Could you check a few things on this model? Use its own coordinates, in mm. Face numbers are marked on the shaded views. A direction names the side the tool comes from. Round coordinates to 2 decimals unless told otherwise and drop trailing zeros. Loops run counter-clockwise (first coordinate to the right, second up) from the corner with the lowest first, then second, coordinate; pieces in that order, holes last. Notation, with made-up numbers: (59.5, -22.75) - (65.5, -22.75) arc R17 ccw to (65.5, 1.25) - close; hole circle Ø5 at (-5, 82.5). An arc over 180 degrees is marked (long way). Put each result on its own line as item: value. Start each with the question number.
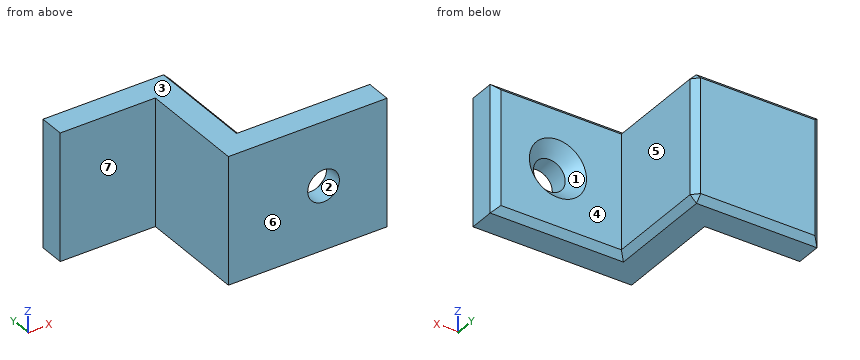
from build123d import *

# Parameters (mm, degrees)
PAD_DEPTH       = 20
SKETCH001_R     = 2.5
POCKET_DEPTH    = 5.001
CHAMFER_SIZE    = 2
CHAMFER001_SIZE = 1


with BuildPart() as part:
    # Sketch → Pad (new body)
    with BuildSketch(Plane.XY):
        Polygon((0, 0), (-25, 0), (-25, 17), (-40, 17), (-40, 22), (-20, 22), (-20, 5), (0, 5), align=None)
    extrude(amount=PAD_DEPTH)

    # Sketch001 (on Face7 of Pad) → Pocket (cut, through all)
    with BuildSketch(Plane(origin=(0, 5, 0), x_dir=(-1, 0, 0), z_dir=(0, 1, 0))):
        with Locations((10, 10)):
            Circle(SKETCH001_R)
    extrude(amount=-POCKET_DEPTH, mode=Mode.SUBTRACT)

    # Chamfer
    chamfer_edges = [part.edges().sort_by_distance(p)[0] for p in [
        (-7.5, 5, 10),
    ]]
    chamfer(chamfer_edges, length=CHAMFER_SIZE)

    # Chamfer001
    chamfer001_edges = [part.edges().sort_by_distance(p)[0] for p in [
        (-10, 5, 0),
        (0, 5, 10),
        (-10, 5, 20),
        (-30, 22, 20),
        (-40, 22, 10),
        (-30, 22, 0),
        (-20, 13.5, 0),
        (-20, 13.5, 20),
        (-20, 22, 10),
    ]]
    chamfer(chamfer001_edges, length=CHAMFER001_SIZE)


solid = part.part
Item 1: Suppose I cut it at A-A, the plane z = 10. List the corners of the cut face in (x, y) for me, then the cut area to 4 significant figures.
Item 2: I need wall thicknesses on line 1 (Z direction, x = -10, y = 1.55); line 2 (X direction, y = 18, z = 8.5); line 3 (Y direction, x = -19, z = 19). Which ranges of each line are inside material? Lowest first, please. Write a range as from..to.
Item 3: On a 3-axis mill with a long thin cutter (end or side, diameter ignored), from which of +Z, -Z, +X, -X, +Y, -Y can I reach the whole of each face in a straight line? I mean the marked faces 5, 6 and 7. Say none if no direction works.
Item 4: Suppose I cut it at D-D, the plane x = -3. List the corners of the cut face in (y, z) for me.
Item 5: Suppose I cut it at B-B, the plane y = 4.5. List the corners of the cut face in (x, z) for me.
Item 6: Suppose I cut it at C-C, the plane x = -10. List the corners of the cut face in (y, z) for me.
Item 7: Thinking about a two-plate mould opening in Z: for the marked faces 1, 2, 3 and 4, which applies, released by +Z, released by -Z, zero draft, split by the parting line, or undercut?
Item 8: Will these pins go through, and if not, where does the flat tip stop? P1, Ø6, axis at x = -6, y = 10, coming from the +Z side; P2, Ø9, axis at x = -12.5, z = 11, coming from the +Y side; P3, Ø8, axis at x = -10, z = 10, coming from the +Y side; P4, Ø1, axis at y = 5, z = 6.5, coming from the +X side.
Numbers:
1. outline: (-40, 17) - (-25, 17) - (-25, 0) - (-12.5, 0) - (-12.5, 3) - (-14.5, 5) - (-20, 5) - (-20, 21) - (-21, 22) - (-39, 22) - (-40, 21) - close; (-7.5, 0) - (0, 0) - (0, 4) - (-1, 5) - (-5.5, 5) - (-7.5, 3) - close
1. area: 254.5 mm^2
2. line 1: 0..7.5, 12.5..20
2. line 2: -40..-20
2. line 3: 0..5
3. face 5: +Z, -Z, +X, +Y
3. face 6: +Z, -Z, +X, -X, -Y
3. face 7: +Z, -Z, -X, -Y
4. outline: (0, 0) - (4, 0) - (5, 1) - (5, 19) - (4, 20) - (0, 20) - close
5. outline: (-25, 0) - (-21, 0) - (-20.5, 0.5) - (-0.5, 0.5) - (-0.5, 19.5) - (-20.5, 19.5) - (-21, 20) - (-25, 20) - close; hole circle Ø8 at (-10, 10)
6. outline: (0, 0) - (4, 0) - (5, 1) - (5, 5.5) - (3, 7.5) - (0, 7.5) - close; (0, 12.5) - (3, 12.5) - (5, 14.5) - (5, 19) - (4, 20) - (0, 20) - close
7. face 1: undercut
7. face 2: undercut
7. face 3: released by +Z
7. face 4: zero draft
8. P1: through
8. P2: y = 5
8. P3: y = 4.5
8. P4: x = -0.5
